The listing builds one solid part. Answer for the finished solid, in the listing's coordinates (mm). A direction names the side the tool comes from. Round coordinates to 2 decimals unless told otherwise and drop trailing zeros. Order: outer loops, then holes, each group sorted by start corner. A loop starts at its lowest first (then second) coordinate and runs counter-clockwise, first axis right, second up. Notation, with made-up numbers: (14.5, 54) -> (32.5, 54) arc R18 cw to (32.5, 84) -> close; hole circle Ø1 at (-28.75, 48). An arc over 180 degrees is marked (long way). Answer in a Markdown table with one row per item. Add a question column.
```python
from build123d import *

# Parameters (mm, degrees)
ESQUISSE2_W                             = 404
ESQUISSE2_H                             = 50
T_LE_DE_BASE_PLI_E1_DEPTH               = 3
T_LE_PLI_E_SUR_AR_TE1_STRIP_W           = 18
T_LE_PLI_E_SUR_AR_TE1_STRIP_H           = 3
T_LE_PLI_E_SUR_AR_TE1_STRIP_CUT_DEPTH   = 404
T_LE_PLI_E_SUR_AR_TE1_STRIP_2_W         = 18
T_LE_PLI_E_SUR_AR_TE1_STRIP_2_H         = 3
T_LE_PLI_E_SUR_AR_TE1_STRIP_CUT_2_DEPTH = 404
T_LE_PLI_E_SUR_AR_TE1_DEPTH             = 404
T_LE_PLI_E_SUR_AR_TE1_BEND_DEPTH        = 404


# Sheet-metal steps are written as plain solids
with BuildPart() as part:
    # Esquisse2 → Tôle de base pliée1 (new body)
    with BuildSketch(Plane(origin=(0, 0, 0), x_dir=(1, 0, 0), z_dir=(0, 1, 0))):
        with Locations((202, 25)):
            Rectangle(ESQUISSE2_W, ESQUISSE2_H)
    extrude(amount=-T_LE_DE_BASE_PLI_E1_DEPTH)

    # Tôle pliée sur arête1 strip (across the edge) → Tôle pliée sur arête1 strip cut (cut)
    with BuildSketch(Plane(origin=(0, 0, 0), x_dir=(0, 0, -1), z_dir=(1, 0, 0))):
        with Locations((-3, -1.5)):
            Rectangle(T_LE_PLI_E_SUR_AR_TE1_STRIP_W, T_LE_PLI_E_SUR_AR_TE1_STRIP_H)
    extrude(amount=T_LE_PLI_E_SUR_AR_TE1_STRIP_CUT_DEPTH, mode=Mode.SUBTRACT)

    # Tôle pliée sur arête1 strip 2 (across the edge) → Tôle pliée sur arête1 strip cut 2 (cut)
    with BuildSketch(Plane(origin=(404, 0, -50), x_dir=(0, 0, 1), z_dir=(-1, 0, 0))):
        with Locations((-3, -1.5)):
            Rectangle(T_LE_PLI_E_SUR_AR_TE1_STRIP_2_W, T_LE_PLI_E_SUR_AR_TE1_STRIP_2_H)
    extrude(amount=T_LE_PLI_E_SUR_AR_TE1_STRIP_CUT_2_DEPTH, mode=Mode.SUBTRACT)

    # Tôle pliée sur arête1 section (across the edge) → Tôle pliée sur arête1 (add)
    with BuildSketch(Plane(origin=(0, 0, 0), x_dir=(0, 0, -1), z_dir=(1, 0, 0))):
        with BuildLine():
            Line((0, 3), (0, 12))
            Line((0, 12), (3, 12))
            Line((3, 12), (3, 3))
            ThreePointArc((3, 3), (3.878679656, 0.878679656), (6, 0))
            Line((6, 0), (6, -3))
            ThreePointArc((6, -3), (1.757359313, -1.242640687), (0, 3))
        make_face()
    extrude(amount=T_LE_PLI_E_SUR_AR_TE1_DEPTH)

    # Tôle pliée sur arête1 section 2 (across the edge) → Tôle pliée sur arête1 bend (add)
    with BuildSketch(Plane(origin=(404, 0, -50), x_dir=(0, 0, 1), z_dir=(-1, 0, 0))):
        with BuildLine():
            Line((0, 3), (0, 12))
            Line((0, 12), (3, 12))
            Line((3, 12), (3, 3))
            ThreePointArc((3, 3), (3.878679656, 0.878679656), (6, 0))
            Line((6, 0), (6, -3))
            ThreePointArc((6, -3), (1.757359313, -1.242640687), (0, 3))
        make_face()
    extrude(amount=T_LE_PLI_E_SUR_AR_TE1_BEND_DEPTH)


solid = part.part
```
1. For faces 1 (the flat face through (199, 0, -25)), 2 (the flat face through (404, -1, -25)), determine the directions among +Z, -Z, +X, -X, +Y, -Y from which every point of the face is accessible in a straight line to the end or side of a thin tool.
2. Each of these flat-tipped pins is pushed along its axis until it touches: pin 1 (10 mm diameter, centred on x = 120.5, z = -30.5, fed in from +Y); pin 2 (2 mm diameter, centred on x = 224, y = 1, fed in from +Z). Where does it stop, or does it pass through?
3. The part is cut by section A-A (y = 7). Give the vertices of the cut face in (x, z).
4. Straight lines are drawn through the part: line 1 along Z through (x, y) = (75, 7.5); line 2 along Y through (x, z) = (66.5, -26); line 3 along Z through (x, y) = (190, 2). For each, find the intervals that lie inside material, in ascending order.
5. The part is cut by section C-C (z = -22). Give the vertices of the cut face in (x, y).
6. The part is cut by section B-B (x = 57). Give the vertices of the cut face in (y, z).
Report:
| question | item | result |
|---|---|---|
| 1 | face 1 | +X, -X, +Y |
| 1 | face 2 | +Z, -Z, +X, +Y, -Y |
| 2 | pin 1 | stops at y = 0 |
| 2 | pin 2 | stops at z = -0.08 |
| 3 | outline | (0, -50) -> (404, -50) -> (404, -47) -> (0, -47) -> close; (0, -3) -> (404, -3) -> (404, 0) -> (0, 0) -> close |
| 4 | line 1 | z = -50 to -47, -3 to 0 |
| 4 | line 2 | y = -3 to 0 |
| 4 | line 3 | z = -49.92 to -46.83, -3.17 to -0.08 |
| 5 | outline | (0, -3) -> (404, -3) -> (404, 0) -> (0, 0) -> close |
| 6 | outline | (-3, -44) arc R6 ccw to (3, -50) -> (12, -50) -> (12, -47) -> (3, -47) arc R3 cw to (0, -44) -> (0, -6) arc R3 cw to (3, -3) -> (12, -3) -> (12, 0) -> (3, 0) arc R6 ccw to (-3, -6) -> close |
